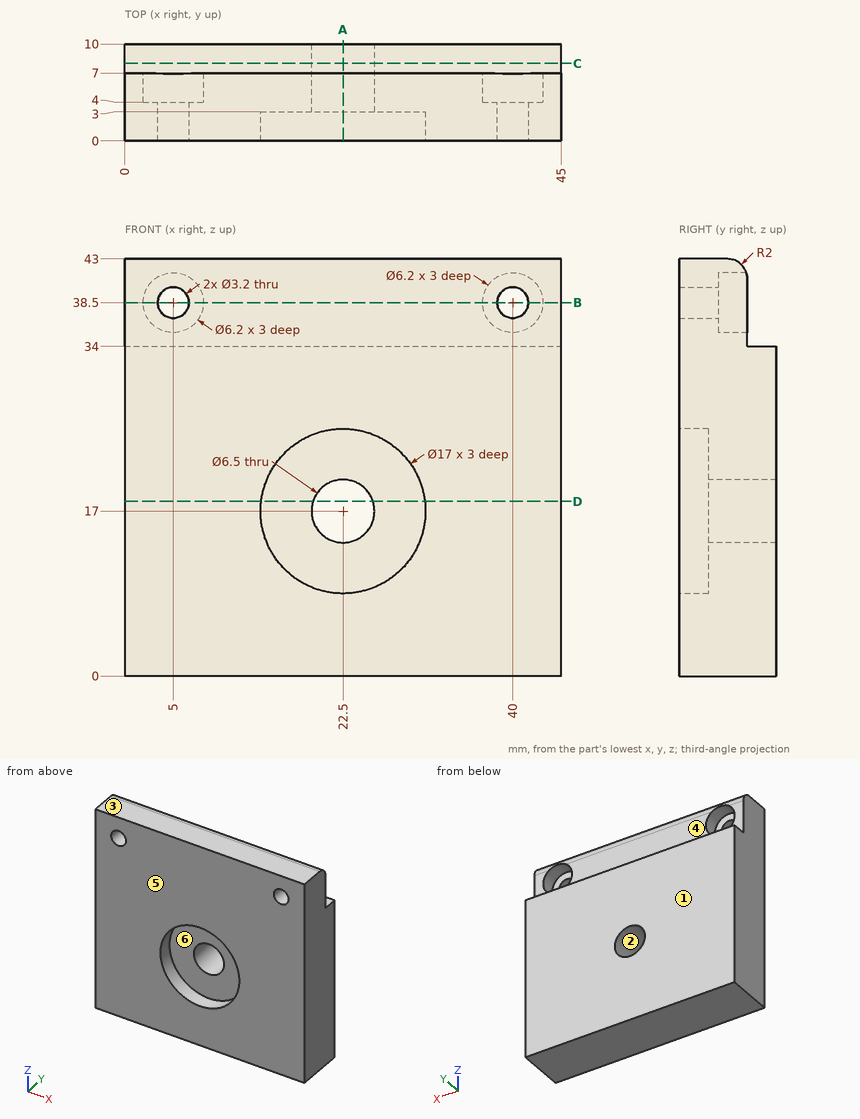
Geometry: see drawing. Coordinates: mm, zero at the bounding-box minimum. A direction names the side the tool comes from. Give positions to 0.01 mm unless a question says otherwise; leave off trailing zeros. Write each loop counter-clockwise with the first axis right and the second up, starting at its lowest first coordinate (ties: lowest second). Pieces come first, ordered by that corner, then holes. Notation, with made-up numbers: M 15.5,-25.75 L 27.5,-25.75 A21 ccw 27.5,10.25 Z; hole C -2.75,17 d7. An arc over 180 degrees is marked long. Answer in a Markdown table with one row per item. Add a question column.
(1) Ray query, line 1 (X direction, y = 6.3, z = 38.5); line 2 (X direction, y = 2.7, z = 38.5); line 3 (Z direction, x = 5, y = 2.75). Return the intervals inside material, ascending.
(2) Section C-C on y = 8. Return loops of the section in (x, z), and give its area (3 significant figures).
(3) Reachability of the marked faces 4, 5 and 6 from +Z, -Z, +X, -X, +Y, -Y: full face, straight path, thin tool, end or side. Return the list, or none.
(4) First-contact query: pin 1 (1.9 mm diameter, centred on x = 5, z = 39.5, fed in from +Y); pin 2 (0.9 mm diameter, centred on x = 21, y = 8.5, fed in from +Z); pin 3 (3.5 mm diameter, centred on x = 17.5, z = 38.5, fed in from +Y). Flat tips, straight axial feed; report the tip coordinate or a pass-through.
(5) Section A-A on x = 22.5. Return loops of the section in (y, z), and give its area (3 significant figures).
(6) Mould query, pull axis Z, two halves, no side actions, for the marked faces 1, 2 and 3. Classes: +Z half, -Z half, draft (parallel to the pull), parting line (faces both ways), or undercut.
(7) Section D-D on z = 18. Return loops of the section in (x, y).
(8) Section B-B on z = 38.5. Return loops of the section in (x, y), and give its area (3 significant figures).
Result set:
| question | item | result |
|---|---|---|
| 1 | line 1 | x = 0 to 1.9, 8.1 to 36.9, 43.1 to 45 |
| 1 | line 2 | x = 0 to 3.4, 6.6 to 38.4, 41.6 to 45 |
| 1 | line 3 | z = 0 to 36.9, 40.1 to 43 |
| 2 | outline | M 0,0 L 45,0 L 45,34 L 0,34 Z; hole C 22.5,17 d6.5 |
| 2 | area | 1,500 mm^2 |
| 3 | face 4 | +Z, +X, -X, +Y |
| 3 | face 5 | +Z, -Z, +X, -X, -Y |
| 3 | face 6 | -Y |
| 4 | pin 1 | stops at y = 4 |
| 4 | pin 2 | stops at z = 34 |
| 4 | pin 3 | stops at y = 7 |
| 5 | outline | M 0,0 L 10,0 L 10,13.75 L 3,13.75 L 3,8.5 L 0,8.5 Z; M 0,25.5 L 3,25.5 L 3,20.25 L 10,20.25 L 10,34 L 7,34 L 7,41 A2 ccw 5,43 L 0,43 Z |
| 5 | area | 306 mm^2 |
| 6 | face 1 | draft |
| 6 | face 2 | undercut |
| 6 | face 3 | +Z half |
| 7 | outline | M 0,0 L 14.06,0 L 14.06,3 L 19.41,3 L 19.41,10 L 0,10 Z; M 25.59,3 L 30.94,3 L 30.94,0 L 45,0 L 45,10 L 25.59,10 Z |
| 8 | outline | M 0,0 L 3.4,0 L 3.4,4 L 1.9,4 L 1.9,7 L 0,7 Z; M 6.6,0 L 38.4,0 L 38.4,4 L 36.9,4 L 36.9,7 L 8.1,7 L 8.1,4 L 6.6,4 Z; M 41.6,0 L 45,0 L 45,7 L 43.1,7 L 43.1,4 L 41.6,4 Z |
| 8 | area | 252 mm^2 |
